Can you work these out from the model? Positions are in its coordinate system, mm. A direction names the side the tool comes from. Give positions to 0.01 mm unless a question says otherwise; leave off trailing zeros. Write each loop counter-clockwise with the first axis right and the second up, starting at its lowest first coordinate (ties: lowest second). Pieces come first, ordered by that corner, then holes.
```python
from build123d import *

# Parameters (mm, degrees)
ESBO_O1_W                = 100
ESBO_O1_H                = 110
RESSALTO_EXTRUS_O1_DEPTH = 18
ESBO_O2_W                = 18
ESBO_O2_H                = 18
RESSALTO_EXTRUS_O2_DEPTH = 10
ESBO_O3_R                = 4.15
CORTE_EXTRUS_O1_DEPTH    = 101


with BuildPart() as part:
    # Esboço1 → Ressalto-extrusão1 (new body)
    with BuildSketch(Plane.XY):
        Rectangle(ESBO_O1_W, ESBO_O1_H)
    extrude(amount=RESSALTO_EXTRUS_O1_DEPTH)

    # Esboço2 → Ressalto-extrusão2 (add)
    with BuildSketch(Plane(origin=(0, 0, 0), x_dir=(-1, 0, 0), z_dir=(0, 0, -1))):
        with Locations((-25, -25)):
            Rectangle(ESBO_O2_W, ESBO_O2_H)
        with Locations((25, -25)):
            Rectangle(ESBO_O2_W, ESBO_O2_H)
        with Locations((-25, 25)):
            Rectangle(ESBO_O2_W, ESBO_O2_H)
        with Locations((25, 25)):
            Rectangle(ESBO_O2_W, ESBO_O2_H)
    extrude(amount=RESSALTO_EXTRUS_O2_DEPTH)

    # Esboço3 → Corte-extrusão1 (cut, through all)
    with BuildSketch(Plane.ZY.offset(50)):
        with Locations((12, 45)):
            Circle(ESBO_O3_R)
        with Locations((12, -45)):
            Circle(ESBO_O3_R)
    extrude(amount=-CORTE_EXTRUS_O1_DEPTH, mode=Mode.SUBTRACT)


solid = part.part
```
1) For pin 1 Ø8 at (x, z) = (25, -7) entering from -Y; pin 2 Ø1.5 at (x, y) = (33.5, 12.5) entering from -Z; pin 3 Ø5 at (y, z) = (22.5, -3) entering from +X, each with a flat end and sliding along its axis, tell me the tip position at first contact or that it passes through.
Values follow:
pin 1: stops at y = -34
pin 2: stops at z = 0
pin 3: stops at x = 34
2) For faces 4 (the face through (-34, 25, -5)), 5 (the face through (-25, 16, -5)), 6 (the face through (-25, 34, -5)), 7 (the face through (-16, -25, -5)), 8 (the face through (34, -25, -5)), which set-ups out of +Z, -Z, +X, -X, +Y, -Y let a thin tool reach every point of the face, with its end or its side?
Values follow:
face 4: -Z, -X, +Y, -Y
face 5: -Z, +X, -X
face 6: -Z, +X, -X, +Y
face 7: -Z, +Y, -Y
face 8: -Z, +X, +Y, -Y
3) Please list where these lines run through material, in increasing order: L1, parallel to Y at x = 10, z = 12; L2, parallel to Y at x = -33, z = -5; L3, parallel to Z at x = -46, y = 44.5.
Values follow:
L1: y = -55 to -49.15, -40.85 to 40.85, 49.15 to 55
L2: y = -34 to -16, 16 to 34
L3: z = 0 to 7.88, 16.12 to 18
4) If we mould it in two halves opening along X, with no side actions, what happens to faces 1 (the face through (25, 25, -10)), 2 (the face through (-34, -25, -5)), 3 (the face through (-16, 25, -5))? For each: +X half, -X half, draft (parallel to the pull), parting line (faces both ways), or undercut.
Values follow:
face 1: draft
face 2: -X half
face 3: undercut
5) Suppose I cut it at D-D on z = 12. Write out the boundary of the cut face in (x, y), plus the area to 3 significant figures.
Values follow:
outline: (-50, -55) - (50, -55) - (50, -49.15) - (-50, -49.15) - close; (-50, -40.85) - (50, -40.85) - (50, 40.85) - (-50, 40.85) - close; (-50, 49.15) - (50, 49.15) - (50, 55) - (-50, 55) - close
area: 9,340 mm2
6) Suppose I cut it at A-A on z = -3.25. Write out the boundary of the cut face in (x, y), plus the area to 3 significant figures.
Values follow:
outline: (-34, -34) - (-16, -34) - (-16, -16) - (-34, -16) - close; (-34, 16) - (-16, 16) - (-16, 34) - (-34, 34) - close; (16, -34) - (34, -34) - (34, -16) - (16, -16) - close; (16, 16) - (34, 16) - (34, 34) - (16, 34) - close
area: 1,300 mm2
7) Suppose I cut it at C-C on y = 45. Write out the boundary of the cut face in (x, z), plus the area to 3 significant figures.
Values follow:
outline: (-50, 0) - (50, 0) - (50, 7.85) - (-50, 7.85) - close; (-50, 16.15) - (50, 16.15) - (50, 18) - (-50, 18) - close
area: 970 mm2
8) Suppose I cut it at B-B on x = -5.5. Write out the boundary of the cut face in (y, z).
Values follow:
outline: (-55, 0) - (55, 0) - (55, 18) - (-55, 18) - close; hole circle Ø8.3 at (-45, 12); hole circle Ø8.3 at (45, 12)
